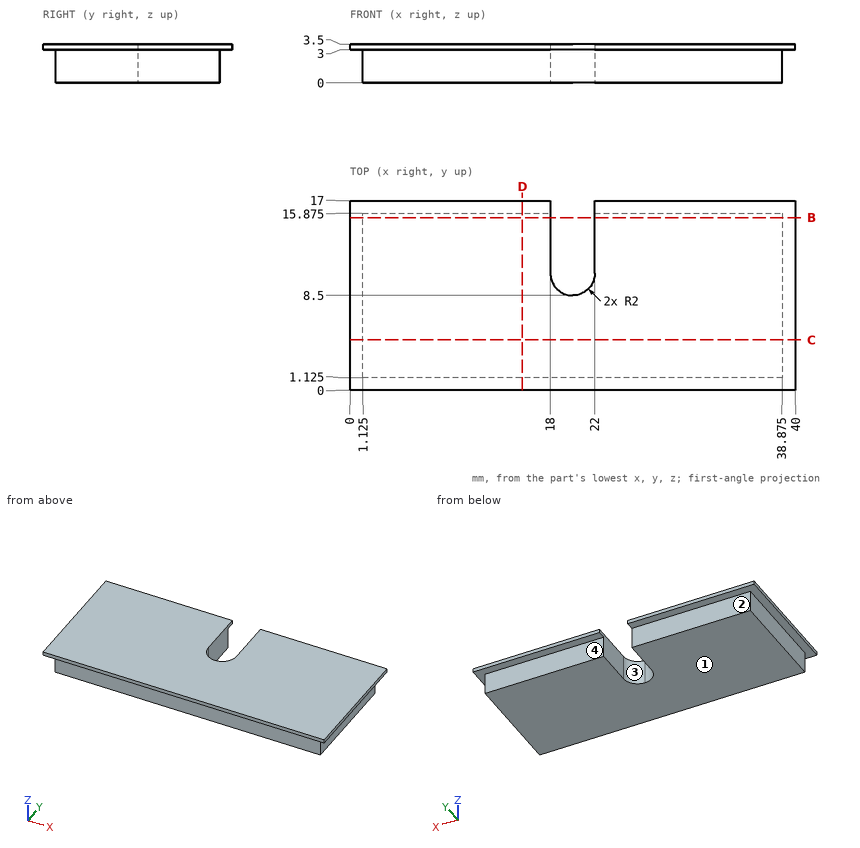
Answer from the drawing. Dimensions are ordinates in mm from the lowest x, y and z of the part. A direction names the side the tool comes from. Coordinates: 2 decimals unless noted, no trailing zeros. Write each loop counter-clockwise with the first axis right and the second up, starting at its lowest first coordinate (ties: lowest second). Pieces come first, ordered by that corner, then holes. Notation, with made-up numbers: M 42.25,23.5 L 68.25,23.5 A14 ccw 68.25,35.5 Z; hole C -26.75,71 d9. An arc over 180 degrees is marked long. Put each result on its own line as item: value. Start each with the question number.
1. For a pull along X with two mould halves and no side action, classify the marked faces 3 and 4 as pulls with the +X half, pulls with the -X half, needs draft (parallel to the pull), parting line crosses it, or undercut.
2. Which of the six approach directions +Z, -Z, +X, -X, +Y, -Y give full straight-line access (tool end or side, diameter ignored) to the marked faces 1 and 2?
3. A cutting plane is placed at C-C on y = 4.5. Write down the section's boundary in (x, z) (3 decimals).
4. Flat-ended cylindrical pins translate along their axes: P1, Ø1.5, axis at y = 4.5, z = 2, coming from the +X side (3 decimals); P2, Ø1.5, axis at x = 27, z = 2, coming from the +Y side (3 decimals). Find the tip coordinate at first contact, or state that the pin passes through.
5. Consider line 1 (X direction, y = 11.5, z = 1.1) (3 decimals); line 2 (X direction, y = 11.5, z = 3.1); line 3 (Y direction, x = 34, z = 0.6) (3 decimals). Determine where each line is inside the solid, lowest interval first. Write a range as from..to.
6. A cutting plane is placed at B-B on y = 15.5. Write down the section's boundary in (x, z) (3 decimals), then the cut area to 3 significant figures.
7. A cutting plane is placed at D-D on x = 15.5. Write down the section's boundary in (y, z) (3 decimals).
Resolved:
1. face 3: undercut
1. face 4: needs draft
2. face 1: -Z, +X, -X, +Y, -Y
2. face 2: -Z, +X, -X, +Y
3. outline: M 0,3 L 1.125,3 L 1.125,0 L 38.875,0 L 38.875,3 L 40,3 L 40,3.5 L 0,3.5 Z
4. P1: stops at x = 38.875
4. P2: stops at y = 15.875
5. line 1: x = 1.125..18, 22..38.875
5. line 2: x = 0..18, 22..40
5. line 3: y = 1.125..15.875
6. outline: M 0,3 L 1.125,3 L 1.125,0 L 18,0 L 18,3.5 L 0,3.5 Z; M 22,0 L 38.875,0 L 38.875,3 L 40,3 L 40,3.5 L 22,3.5 Z
6. area: 119 mm2
7. outline: M 0,3 L 1.125,3 L 1.125,0 L 15.875,0 L 15.875,3 L 17,3 L 17,3.5 L 0,3.5 Z
